```python
from build123d import *

# Parameters (mm, degrees)
SKETCH1_W           = 2300
SKETCH1_H           = 900
SKETCH1_W_2         = 525
SKETCH1_H_2         = 800
SKETCH1_W_3         = 492.389580631
SKETCH1_W_4         = 507.610419369
BOSS_EXTRUDE1_DEPTH = 60
SKETCH2_W           = 42.389580631
SKETCH2_H           = 50
SKETCH2_W_2         = 57.610419369
BOSS_EXTRUDE2_DEPTH = 1
SKETCH4_W           = 50
SKETCH4_H           = 50.463593603
BOSS_EXTRUDE4_DEPTH = 1
SKETCH5_W           = 44.216514846
SKETCH5_H           = 50
BOSS_EXTRUDE5_DEPTH = 1
SKETCH6_W           = 42.447812038
SKETCH6_H           = 50
BOSS_EXTRUDE6_DEPTH = 1
BOSS_EXTRUDE7_DEPTH = 1


with BuildPart() as part:
    # Sketch1 → Boss-Extrude1 (new body)
    with BuildSketch(Plane.XY):
        Rectangle(SKETCH1_W, SKETCH1_H)
        with Locations((-287.5, 0)):
            Rectangle(SKETCH1_W_2, SKETCH1_H_2, mode=Mode.SUBTRACT)
        with Locations((287.5, 0)):
            Rectangle(SKETCH1_W_2, SKETCH1_H_2, mode=Mode.SUBTRACT)
        with Locations((846.194790316, 0)):
            Rectangle(SKETCH1_W_3, SKETCH1_H_2, mode=Mode.SUBTRACT)
        with Locations((-853.805209685, 0)):
            Rectangle(SKETCH1_W_4, SKETCH1_H_2, mode=Mode.SUBTRACT)
    extrude(amount=BOSS_EXTRUDE1_DEPTH)

    # Sketch2 → Boss-Extrude2 (add)
    with BuildSketch(Plane.XY.offset(60)):
        with Locations((-1128.805209684, -425)):
            Rectangle(SKETCH2_W, SKETCH2_H)
        with Locations((1121.194790316, -425)):
            Rectangle(SKETCH2_W_2, SKETCH2_H)
    extrude(amount=BOSS_EXTRUDE2_DEPTH)

    # Sketch4 → Boss-Extrude4 (add)
    with BuildSketch(Plane(origin=(0, 0, 0), x_dir=(-1, 0, 0), z_dir=(0, 0, -1))):
        with Locations((0, -425.231796802)):
            Rectangle(SKETCH4_W, SKETCH4_H)
    extrude(amount=BOSS_EXTRUDE4_DEPTH)

    # Sketch5 → Boss-Extrude5 (add)
    with BuildSketch(Plane(origin=(0, 0, 0), x_dir=(-1, 0, 0), z_dir=(0, 0, -1))):
        with Locations((-181.41, -425)):
            Rectangle(SKETCH5_W, SKETCH5_H)
    extrude(amount=BOSS_EXTRUDE5_DEPTH)

    # Sketch6 → Boss-Extrude6 (add)
    with BuildSketch(Plane(origin=(0, 0, 0), x_dir=(-1, 0, 0), z_dir=(0, 0, -1))):
        with Locations((223.59, -425)):
            Rectangle(SKETCH6_W, SKETCH6_H)
    extrude(amount=BOSS_EXTRUDE6_DEPTH)

    # Sketch7 → Boss-Extrude7 (add)
    with BuildSketch(Plane(origin=(0, 0, 0), x_dir=(-1, 0, 0), z_dir=(0, 0, -1))):
        Polygon((740.20473979, -400), (763.59, -400), (786.97526021, -400), (786.97526021, -450), (763.59, -450), (740.20473979, -450), align=None)
    extrude(amount=BOSS_EXTRUDE7_DEPTH)


solid = part.part
```
Source: CAD feature listing. Evaluate the final solid. Frame: model axes, mm. A direction names the side the tool comes from. Coordinates: 2 decimals unless noted, no trailing zeros. Write each loop counter-clockwise with the first axis right and the second up, starting at its lowest first coordinate (ties: lowest second). Pieces come first, ordered by that corner, then holes. Notation, with made-up numbers: (83.25, 37) -> (127.25, 37) arc R20 cw to (127.25, 54) -> close; hole circle Ø7 at (52, 46). An arc over 180 degrees is marked (long way). Return JSON: item names as keys, results as strings. Group by question number.
1) Set-up query: faces 4 (the face through (1121, -425, 61)), 5 (the face through (-1107.61, -6, 30)). Return all of +Z, -Z, +X, -X, +Y, -Y with unobstructed straight access to the full face (end or side cutting, diameter ignored); none if empty.
2) Ray query, line 1 along X through (y, z) = (-364, 6); line 2 along Y through (x, z) = (412.5, 38); line 3 along Z through (x, y) = (-561.5, 256). Return the intervals inside material, ascending.
3) Section query C-C, the plane z = 28.5. Return loops of the section in (x, y), plus the area to 3 significant figures.
4) Section query A-A, the plane y = -250.5. Return loops of the section in (x, z).
5) Contact query for flat-ended pins moving along their axis: P1, Ø0.5, axis at x = -10, z = -0.5, coming from the +Y side; P2, Ø18, axis at x = -197, z = 19, coming from the -Y side; P3, Ø4, axis at x = 582.5, y = -314.5, coming from the +Z side. Output: stop coordinate, or through.
6) Mould query, pull axis Y, two halves, no side actions, for faces 1 (the face through (-25, -6, 30)), 2 (the face through (182, -425, -1)), 3 (the face through (-16, -450, 30)). Classes: +Y half, -Y half, draft (parallel to the pull), parting line (faces both ways), or undercut.
7) Section query B-B, the plane x = -498.5. Return loops of the section in (y, z), plus the area to 3 significant figures.
From the geometry:
{
 "1": {"face 4": "+Z, +X, -X, +Y, -Y", "face 5": "+Z, -Z"},
 "2": {"line 1": "-1150 to -1107.61, -600 to -550, -25 to 25, 550 to 600, 1092.39 to 1150", "line 2": "-450 to -400, 400 to 450", "line 3": "0 to 60"},
 "3": {"outline": "(-1150, -450) -> (1150, -450) -> (1150, 450) -> (-1150, 450) -> close; hole (-1107.61, -400) -> (-600, -400) -> (-600, 400) -> (-1107.61, 400) -> close; hole (-550, -400) -> (-25, -400) -> (-25, 400) -> (-550, 400) -> close; hole (25, -400) -> (550, -400) -> (550, 400) -> (25, 400) -> close; hole (600, -400) -> (1092.39, -400) -> (1092.39, 400) -> (600, 400) -> close", "area": "430,000 mm²"},
 "4": {"outline": "(-1150, 0) -> (-1107.61, 0) -> (-1107.61, 60) -> (-1150, 60) -> close; (-600, 0) -> (-550, 0) -> (-550, 60) -> (-600, 60) -> close; (-25, 0) -> (25, 0) -> (25, 60) -> (-25, 60) -> close; (550, 0) -> (600, 0) -> (600, 60) -> (550, 60) -> close; (1092.39, 0) -> (1150, 0) -> (1150, 60) -> (1092.39, 60) -> close"},
 "5": {"P1": "y = -400", "P2": "y = -450", "P3": "z = 60"},
 "6": {"face 1": "undercut", "face 2": "draft", "face 3": "-Y half"},
 "7": {"outline": "(-450, 0) -> (-400, 0) -> (-400, 60) -> (-450, 60) -> close; (400, 0) -> (450, 0) -> (450, 60) -> (400, 60) -> close", "area": "6,000 mm²"}
}
